Build history of the part. All positions in model axes, mm. A direction names the side the tool comes from. Round coordinates to 2 decimals unless told otherwise and drop trailing zeros. Order: outer loops, then holes, each group sorted by start corner. A loop starts at its lowest first (then second) coordinate and runs counter-clockwise, first axis right, second up. Notation, with made-up numbers: M 34.5,38 L 92.5,38 A18 cw 92.5,50 Z; hole C 67,34.25 d11. An arc over 180 degrees is marked long. One line per item, written item: value. Start each with the question number.
Item 1: Band-saw the part on C-C, the plane z = 10.75. Write the cut outline in (x, y), then the cut area to 3 significant figures.
Item 2: Two-plate mould, pull along X, no slides. Class faces 6 (the flat face through (-14, 3, 3)), 7 (the flat face through (11, 0, 3)), 8 (the cylindrical face through (31.55, 10.85, 13.24)), 9 (the cylindrical face through (-13.483, 2.958, -0.26)): +X half, -X half, draft (parallel to the pull), parting line (faces both ways), or undercut.
Item 3: Band-saw the part on B-B, the plane y = 12. Write the cut outline in (x, z), then the cut area to 3 significant figures.
Item 4: Band-saw the part on D-D, the plane z = -5.25. Write the cut outline in (x, y).
Item 5: Tool access for faces 1 (the flat face through (4, 5, -4)), 2 (the flat face through (13, 15, -2)), 3 (the flat face through (15, 11, -2)), 4 (the flat face through (-15, 3, 0)), 5 (the flat face through (-3, 3, 4)): list every direction of +Z, -Z, +X, -X, +Y, -Y with a clear straight run to the whole face (end or side of a thin tool).
Item 6: Pin check, flat tips, straight feed: pin 1 (6.5 mm diameter, centred on x = -1, y = 4.5, fed in from +Z); pin 2 (12 mm diameter, centred on y = 17, z = 1.5, fed in from +X); pin 3 (10 mm diameter, centred on y = 8.5, z = 7.5, fed in from +X); pin 4 (5 mm diameter, centred on y = 4.5, z = 7.5, fed in from +X). Stop position of each tip, or through.
Item 7: Band-saw the part on A-A, the plane x = -4. Write the cut outline in (y, z), then the cut area to 3 significant figures.
Item 8: Probe L1, parallel to X at y = 2.8, z = 0; L2, parallel to X at y = 19, z = -0.5; L3, parallel to Z at x = 3.5, y = 3.55. List the from-to ranges inside material, lowest first.
Autodesk Inventor part; units mm, degrees
ref_plane "YZ Plane" through (0, 0, 0) normal (1, 0, 0) x (0, 1, 0)
ref_plane "XZ Plane" through (0, 0, 0) normal (0, 1, 0) x (-1, 0, 0)
ref_plane "XY Plane" through (0, 0, 0) normal (0, 0, 1) x (1, 0, 0)
sketch "Sketch1" plane through (0, 0, 0) normal (0, 1, 0) x (-1, 0, 0)
  line L0 (15, 4) -> (-15, 4)
  line L1 (-15, 4) -> (-15, -4)
  line L2 (-15, -4) -> (15, -4)
  line L3 (15, -4) -> (15, 4)
  line L4 (15, 4) -> (-15, -4) construction
  line L5 (-15, 4) -> (15, -4) construction
  point P0 (0, 0)
  dimension "d0" = 8
  dimension "d1" = 30
extrude "Extrusion1" add sketch "Sketch1" along normal blind 6
sketch "Sketch2" plane through (0, 6, 0) normal (0, 1, 0) x (1, 0, 0)
  line L0 (15, -4) -> (15, 4)
  line L1 (15, 4) -> (-15, 4)
  line L2 (-15, 4) -> (-15, -4)
  line L3 (-15, -4) -> (15, -4)
  point P0 (0, 0)
  point P1 (-4, 0)
  point P2 (-11.5, 0)
  point P3 (3.5, 0)
  dimension "d4" = 7.5
  dimension "d5" = 11
  dimension "d14" = 7.5
hole "Hole1" at (-4, 6, 0) at (-11.5, 6, 0) at (3.5, 6, 0) direction (0, -1, 0) diameter 4 end through all
sketch "Sketch3" plane through (0, 6, 0) normal (0, 1, 0) x (1, 0, 0)
  line L0 (15, -4) -> (15, 4)
  arc A0 (15, 0) -> (36.7378, 7.0126) centre (27, 0) ccw
  arc A1 (13, 0) -> (38.4773, 8.0169) centre (27, 0) ccw
  line L1 (38.4773, 8.0169) -> (36.7378, 7.0126)
  line L2 (15, 0) -> (15, 4)
  line L3 (15, 4) -> (-15, 4)
  line L4 (13, 4) -> (13, 0)
  point P0 (0, 0)
  dimension "d15" = 2
  dimension "d16" = 0
  dimension "d17" = 60
  dimension "d22" = 12
extrude "Extrusion2" add sketch "Sketch3" along normal blind 16 and the other way blind 6
chamfer "Chamfer1" distance 5 angle 45 2 edges at (13, 6, -2) (13.1467, 6, 2.0212)
chamfer "Chamfer2" distance 2 angle 45 2 edges at (-15, 3, 4) (-15, 3, -4)
chamfer "Chamfer3" distance 4 angle 45 3 edges at (14, 22, -4) (37.6076, 22, -7.5147) (37.6076, 0, -7.5147)
fillet "Fillet1" radius 12 1 edges at (13.5836, 3, 4)
fillet "Fillet2" radius 4 1 edges at (11.865, 8.9761, 5.2631)
properties part number "squirrely_leg"
Output:
1. outline: M 18.03,0 L 21.67,0 L 21.67,22 L 18.03,22 Z; M 32.33,0 L 35.97,0 L 35.97,22 L 32.33,22 Z
1. area: 160 mm²
2. face 6: -X half
2. face 7: draft
2. face 8: parting line
2. face 9: undercut
3. outline: M 13,-4 L 15,-4 L 15,0 A12 cw long 36.74,-7.01 L 38.48,-8.02 A14 ccw long 13,0 Z
3. area: 106 mm²
4. outline: M 37.79,1.95 L 39.98,0.85 L 39.98,21.15 L 37.79,20.05 Z
5. face 1: -Z, -X, +Y, -Y
5. face 2: +Z, -Z, -X, +Y
5. face 3: -Z, +Y, -Y
5. face 4: +Z, -Z, -X, +Y, -Y
5. face 5: +Z, -X, +Y, -Y
6. pin 1: stops at z = 4
6. pin 2: stops at x = 41
6. pin 3: stops at x = 40.77
6. pin 4: stops at x = 40.08
7. outline: M 0,-4 L 6,-4 L 6,-2 L 0,-2 Z; M 0,2 L 6,2 L 6,4 L 0,4 Z
7. area: 24.0 mm²
8. L1: x = -15 to -13.5, -9.5 to -6, -2 to 1.5, 5.5 to 15, 39 to 41
8. L2: x = 13 to 15, 38.99 to 40.99
8. L3: z = -4 to -2, 2 to 4
